```python
from build123d import *

# Parameters (mm, degrees)
SKETCH1_W               = 25
SKETCH1_H               = 30
BOSS_EXTRUDE1_DEPTH     = 1.6
BOSS_EXTRUDE2_DEPTH     = 3
SKETCH3_R               = 7
BOSS_EXTRUDE3_DEPTH     = 3
BOSS_EXTRUDE4_START     = 3
SKETCH4_R               = 7
BOSS_EXTRUDE4_DEPTH     = 3
SKETCH5_R               = 6
BOSS_EXTRUDE5_DEPTH     = 3.5
SKETCH6_R               = 8
BOSS_EXTRUDE6_DEPTH     = 1
SKETCH10_R              = 1.5
CUT_EXTRUDE1_DEPTH      = 2
MIRROR2_COPY_1_SKETCH_R = 1.5
MIRROR2_COPY_1_DEPTH    = 2
SKETCH11_W              = 4.4
SKETCH11_H              = 7.4
BOSS_EXTRUDE7_DEPTH     = 3.2
CUT_EXTRUDE2_DEPTH      = 3
SKETCH13_W              = 7.4
SKETCH13_H              = 0.01
CUT_EXTRUDE3_DEPTH      = 3


with BuildPart() as part:
    # Sketch1 → Boss-Extrude1 (new body)
    with BuildSketch(Plane(origin=(0, 0, 0), x_dir=(1, 0, 0), z_dir=(0, 1, 0))):
        Rectangle(SKETCH1_W, SKETCH1_H)
    extrude(amount=BOSS_EXTRUDE1_DEPTH)

    # Sketch2 → Boss-Extrude2 (add)
    with BuildSketch(Plane(origin=(0, 1.6, 0), x_dir=(1, 0, 0), z_dir=(0, 1, 0))):
        with BuildLine():
            Line((2, -9.8), (2, -7))
            Line((2, -7), (6.5, -7))
            Line((6.5, -7), (6.5, 7))
            Line((6.5, 7), (2, 7))
            Line((2, 7), (2, 9.8))
            ThreePointArc((2, 9.8), (0, 11.4), (-2, 9.8))
            Line((-2, 9.8), (-2, 7))
            Line((-2, 7), (-6.5, 7))
            Line((-6.5, 7), (-6.5, -7))
            Line((-6.5, -7), (-2, -7))
            Line((-2, -7), (-2, -9.8))
            ThreePointArc((-2, -9.8), (0, -11.4), (2, -9.8))
        make_face()
    extrude(amount=BOSS_EXTRUDE2_DEPTH)

    # Sketch3 → Boss-Extrude3 (add)
    with BuildSketch(Plane(origin=(0, 4.6, 0), x_dir=(1, 0, 0), z_dir=(0, 1, 0))):
        Circle(SKETCH3_R)
    extrude(amount=-BOSS_EXTRUDE3_DEPTH)

    # Sketch4 → Boss-Extrude4 (add)
    with BuildSketch(Plane(origin=(0, 4.6, 0), x_dir=(1, 0, 0), z_dir=(0, 1, 0)).offset(BOSS_EXTRUDE4_START)):
        with Locations(Location((0, 0, 0), (0, 0, 270))):
            Circle(SKETCH4_R)
    extrude(amount=-BOSS_EXTRUDE4_DEPTH)

    # Sketch5 → Boss-Extrude5 (add)
    with BuildSketch(Plane(origin=(0, 7.6, 0), x_dir=(1, 0, 0), z_dir=(0, 1, 0))):
        with Locations(Location((0, 0, 0), (0, 0, 270))):
            Circle(SKETCH5_R)
    extrude(amount=BOSS_EXTRUDE5_DEPTH)

    # Sketch6 → Boss-Extrude6 (add)
    with BuildSketch(Plane(origin=(0, 11.1, 0), x_dir=(1, 0, 0), z_dir=(0, 1, 0))):
        with Locations(Location((0, 0, 0), (0, 0, 270))):
            Circle(SKETCH6_R)
    extrude(amount=BOSS_EXTRUDE6_DEPTH)

    # Loft1: read off the stored shape, not the designer's step
    # Loft1: loft between two sections, ruled curve by curve
    loft1_from = [
        Edge.make_bspline([(-7.29329327, 12.1, -3.287533007), (-13.868359284, 12.1, 11.299053534), (0.718227257, 12.1, 17.874119548), (7.29329327, 12.1, 3.287533007), (13.868359284, 12.1, -11.299053534), (-0.718227257, 12.1, -17.874119548), (-7.29329327, 12.1, -3.287533007)], [0, 0, 0, 0, 0.5, 0.5, 0.5, 1, 1, 1, 1], 3, [1, 0.333333333, 0.333333333, 1, 0.333333333, 0.333333333, 1]),
    ]
    loft1_to = [
        Edge.make_bspline([(-4.457852082, 13.1, 0.614454893), (-3.228942297, 13.1, 9.530159057), (5.686761867, 13.1, 8.301249271), (4.457852082, 13.1, -0.614454893), (3.228942297, 13.1, -9.530159057), (-5.686761867, 13.1, -8.301249271), (-4.457852082, 13.1, 0.614454893)], [0, 0, 0, 0, 0.5, 0.5, 0.5, 1, 1, 1, 1], 3, [1, 0.333333333, 0.333333333, 1, 0.333333333, 0.333333333, 1]),
    ]
    loft1 = Solid(Shell([*[Face.make_surface_from_curves(loft1_from[k], loft1_to[k]) for k in range(1)], Face(Wire(loft1_from)), Face(Wire(loft1_to))]))
    add(loft1)

    # Sketch10 → Cut-Extrude1 (cut)
    with BuildSketch(Plane(origin=(0, 1.6, 0), x_dir=(1, 0, 0), z_dir=(0, 1, 0))):
        with Locations((12.5, -12)):
            Circle(SKETCH10_R)
    cut_extrude1 = extrude(amount=-CUT_EXTRUDE1_DEPTH, mode=Mode.SUBTRACT)

    # Mirror1: Cut-Extrude1 across plane
    add(cut_extrude1.mirror(Plane.ZY), mode=Mode.SUBTRACT)

    # Mirror2: Cut-Extrude1 across plane
    add(cut_extrude1.mirror(Plane.XY), mode=Mode.SUBTRACT)

    # Mirror2 copy 1 sketch → Mirror2 copy 1 (cut)
    with BuildSketch(Plane(origin=(0, 1.6, 0), x_dir=(-1, 0, 0), z_dir=(0, 1, 0))):
        with Locations((12.5, -12)):
            Circle(MIRROR2_COPY_1_SKETCH_R)
    extrude(amount=-MIRROR2_COPY_1_DEPTH, mode=Mode.SUBTRACT)

    # Sketch11 → Boss-Extrude7 (add)
    with BuildSketch(Plane(origin=(0, 0, 0), x_dir=(-1, 0, 0), z_dir=(0, -1, 0))):
        with Locations((10.3, 5.5)):
            Rectangle(SKETCH11_W, SKETCH11_H)
    extrude(amount=BOSS_EXTRUDE7_DEPTH)

    # Sketch12 → Cut-Extrude2 (cut)
    with BuildSketch(Plane.ZY.offset(12.5)):
        Polygon((-8.4, -2.7), (-2.6, -2.7), (-2.6, -2.4), (-2.5, -2.4), (-2.5, -1.9), (-2.6, -1.9), (-2.6, -0.5), (-8.4, -0.5), (-8.4, -1.9), (-8.5, -1.9), (-8.5, -2.4), (-8.4, -2.4), align=None)
    extrude(amount=-CUT_EXTRUDE2_DEPTH, mode=Mode.SUBTRACT)

    # Sketch13 → Cut-Extrude3 (cut)
    with BuildSketch(Plane.ZY.offset(12.5)):
        with Locations((-5.5, -0.005)):
            Rectangle(SKETCH13_W, SKETCH13_H)
    extrude(amount=-CUT_EXTRUDE3_DEPTH, mode=Mode.SUBTRACT)


solid = part.part
```
The model under review builds one solid part; all positions refer to its coordinate system, in mm. A direction names the side the tool comes from. Round coordinates to 2 decimals unless told otherwise and drop trailing zeros. Loops run counter-clockwise (first coordinate to the right, second up) from the corner with the lowest first, then second, coordinate; pieces in that order, holes last. Notation, with made-up numbers: (-36, -31.5) -> (-17, -31.5) arc R13 cw to (-17, -21.5) -> close; hole circle Ø5 at (67, 24.5). An arc over 180 degrees is marked (long way). Answer as a JSON object with one key per item and string values. Group by question number.
1) For pin 1 Ø12.5 at (x, z) = (4.5, 7.5) entering from -Y; pin 2 Ø1 at (y, z) = (3, 1.5) entering from +X; pin 3 Ø1.5 at (y, z) = (4, -5) entering from +X; pin 4 Ø3 at (y, z) = (11.5, -10.5) entering from +X, all flat-tipped, find the tip position at first contact; note any pin that passes through.
2) For faces 1 (the face through (-4, 3, -7)), 2 (the face through (2, 7.6, 6)), 3 (the face through (2, 3, -8)), 4 (the face through (-4, 3, 7)), list the 3-axis set-ups (+Z, -Z, +X, -X, +Y, -Y) from which the entire face can be reached by the end or side of a thin tool; tool diameter is ignored.
3) We need section A-A on z = 12. Write out the cut boundary in (x, y), then the cut area to 3 significant figures.
4) For line 1 (X direction, y = 3.75, z = 5.5); line 2 (Y direction, x = 4, z = -8.25); line 3 (Z direction, x = -8.75, y = -1.5), list the stretches that pass through material, from the lowest coordinate up. Write a range as [from, to].
Result set:
{
 "1": {"pin 1": "y = 0", "pin 2": "x = 6.93", "pin 3": "x = 6.5", "pin 4": "through"},
 "2": {"face 1": "-Z, -X", "face 2": "none", "face 3": "-Z, +X", "face 4": "+Z, -X"},
 "3": {"outline": "(-11, 0) -> (11, 0) -> (11, 1.6) -> (-11, 1.6) -> close", "area": "35.2 mm²"},
 "4": {"line 1": "[-6.5, 6.5]", "line 2": "[0, 1.6]", "line 3": "[-9.2, -1.8]"}
}
